Check sheet for the modelled part. Datum: model origin and axes. Units: mm. Face numbers are marked on the shaded views. A direction names the side the tool comes from. Round coordinates to 2 decimals unless told otherwise and drop trailing zeros. Order: outer loops, then holes, each group sorted by start corner. A loop starts at its lowest first (then second) coordinate and runs counter-clockwise, first axis right, second up. Notation, with made-up numbers: (13, 14.25) -> (19, 14.25) arc R21 ccw to (19, 50.25) -> close; hole circle Ø4 at (34, 38). An arc over 180 degrees is marked (long way). Answer as CSV lines item,"result". Start each with the question number.
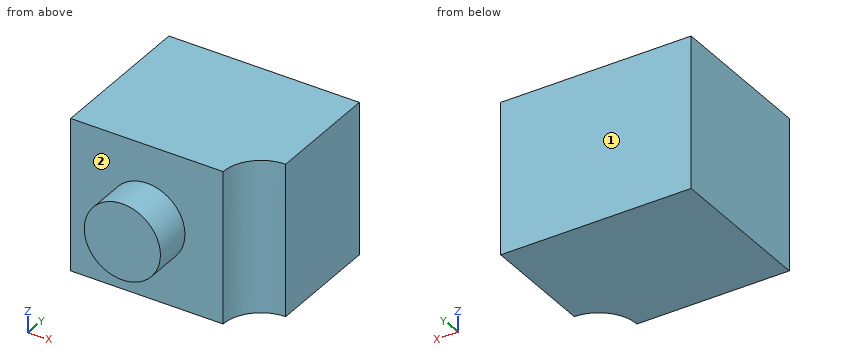
from build123d import *

# Parameters (mm, degrees)
F0_W     = 5
F0_H     = 4
F1_DEPTH = 4
F2_R     = 1
F3_DEPTH = 4.1
F4_R     = 1
F5_DEPTH = 1


with BuildPart() as f1:
    # F0 (on Top) → F1 (new body)
    with BuildSketch(Plane.XY):
        with Locations((21.835487, 15.660429)):
            Rectangle(F0_W, F0_H)
    extrude(amount=F1_DEPTH)

    # F2 (on face) → F3 (cut)
    with BuildSketch(Plane.XY.offset(4)):
        with Locations((24.335487, 13.660429)):
            Circle(F2_R)
    extrude(amount=-F3_DEPTH, mode=Mode.SUBTRACT)

    # F4 (on face) → F5 (join)
    with BuildSketch(Plane.XZ.offset(-13.660429)):
        with Locations((21.335487, 2)):
            Circle(F4_R)
    extrude(amount=F5_DEPTH)


solid = f1.part
1) Material ranges on line 1 along Y through (x, z) = (20.2, 0.3); line 2 along X through (y, z) = (13.7, 3.15); line 3 along X through (y, z) = (13.6, 1.2), recorded low to high.
2) Section check B-B on x = 21.1. Record the cut outline in (y, z).
3) Section check C-C on z = 3.65. Record the cut outline in (x, y), then the cut area to 3 significant figures.
4) Access from +Z, -Z, +X, -X, +Y, -Y to the whole of each face (thin tool, end or side, straight path). Record for the marked faces 1 and 2.
5) Section check D-D on x = 21.9. Record the cut outline in (y, z).
6) Section check A-A on z = 2. Record the cut outline in (x, y).
Solutions:
1,line 1,"y = 13.66 to 17.66"
1,line 2,"x = 19.34 to 23.34"
1,line 3,"x = 20.74 to 21.94"
2,outline,"(12.66, 1.03) -> (13.66, 1.03) -> (13.66, 0) -> (17.66, 0) -> (17.66, 4) -> (13.66, 4) -> (13.66, 2.97) -> (12.66, 2.97) -> close"
3,outline,"(19.34, 13.66) -> (23.34, 13.66) arc R1 cw to (24.34, 14.66) -> (24.34, 17.66) -> (19.34, 17.66) -> close"
3,area,"19.2 mm^2"
4,face 1,"+Z, -Z, +X, -X, +Y"
4,face 2,"-Y"
5,outline,"(12.66, 1.17) -> (13.66, 1.17) -> (13.66, 0) -> (17.66, 0) -> (17.66, 4) -> (13.66, 4) -> (13.66, 2.83) -> (12.66, 2.83) -> close"
6,outline,"(19.34, 13.66) -> (20.34, 13.66) -> (20.34, 12.66) -> (22.34, 12.66) -> (22.34, 13.66) -> (23.34, 13.66) arc R1 cw to (24.34, 14.66) -> (24.34, 17.66) -> (19.34, 17.66) -> close"
